Verification items for the finished model (mm, model axes). Give positions to 0.01 mm unless a question says otherwise; leave off trailing zeros. Order: outer loops, then holes, each group sorted by start corner. A loop starts at its lowest first (then second) coordinate and runs counter-clockwise, first axis right, second up. Notation, with made-up numbers: (85.25, 21.5) -> (112.25, 21.5) arc R25 ccw to (112.25, 48.5) -> close; hole circle Ø2 at (42, 52.5). An arc over 180 degrees is marked (long way). Write each question's results on one line, items separated by ' | '. Start each with the question number.
1. Depth check by flat-ended pin: pin 1 Ø10 at (y, z) = (-15, 9) entering from +X; pin 2 Ø4 at (x, y) = (-12.5, 10.5) entering from -Z; pin 3 Ø10 at (x, z) = (12.5, -0.5) entering from +Y. Enter the tip coordinate at first touch or a pass-through.
2. Material ranges on L1, parallel to Y at x = 0, z = 12.75; L2, parallel to Y at x = 0, z = 7.75; L3, parallel to Y at x = 4.5, z = -2, recorded low to high. Write a range as from..to.
3. Cross-section at D-D, the plane z = -16. Enter the section's corners in (x, y).
4. Cross-section at A-A, the plane x = 0. Enter the section's corners in (y, z).
5. Cross-section at C-C, the plane z = 14.5. Enter the section's corners in (x, y) (1 decimal).
6. Mould release check, pull along Y, two halves, no side actions. Record for faces 1 (the face through (-3.78, -2.9, 9.74)), 2 (the face through (4.4, -2.2, 16.002)): +Y half, -Y half, draft (parallel to the pull), parting line (faces both ways), or undercut.
from build123d import *

# Parameters (mm, degrees)
SKETCH3_W          = 37.025629418
SKETCH3_H          = 29.353652152
CUT_EXTRUDE1_DEPTH = 3.048
SKETCH4_R          = 4.7625
CUT_EXTRUDE2_DEPTH = 12.7


with BuildPart() as part:
    # Sketch1 → Revolve6 (revolve)
    with BuildSketch(Plane(origin=(0, 0, 0), x_dir=(1, 0, 0), z_dir=(0, 1, 0))):
        with BuildLine():
            Line((0, 0), (19.05, 0))
            ThreePointArc((19.05, 0), (0, -19.05), (-19.05, 0))
            Line((-19.05, 0), (0, 0))
        make_face()
    revolve(axis=Axis((-19.05, 0, 0), (1, 0, 0)))

    # Sketch3 → Cut-Extrude1 (cut)
    with BuildSketch(Plane.XY.offset(16.002)):
        Rectangle(SKETCH3_W, SKETCH3_H)
    extrude(amount=CUT_EXTRUDE1_DEPTH, mode=Mode.SUBTRACT)

    # Sketch4 → Cut-Extrude2 (cut)
    with BuildSketch(Plane.XY.offset(16.002)):
        Circle(SKETCH4_R)
    extrude(amount=-CUT_EXTRUDE2_DEPTH, mode=Mode.SUBTRACT)


solid = part.part
Results below:
1) pin 1: stops at x = 14.38 | pin 2: stops at z = -12.56 | pin 3: stops at y = 17.51
2) L1: y = -14.15..-4.76, 4.76..14.15 | L2: y = -17.4..-4.76, 4.76..17.4 | L3: y = -18.4..18.4
3) outline: circle Ø20.68 at (0, 0)
4) outline: (-10.34, 16) arc R19.05 ccw (long way) to (10.34, 16) -> (4.76, 16) -> (4.76, 3.3) -> (-4.76, 3.3) -> (-4.76, 16) -> close
5) outline: circle Ø24.7 at (0, 0); hole circle Ø9.5 at (0, 0)
6) face 1: undercut | face 2: draft
